Here's how the part is built. I have some questions about the finished solid (model axes, mm). Coordinates: 2 decimals unless noted, no trailing zeros. Order: outer loops, then holes, each group sorted by start corner. A loop starts at its lowest first (then second) coordinate and runs counter-clockwise, first axis right, second up. Notation, with made-up numbers: M 58.5,38 L 93.5,38 A12 cw 93.5,58 Z; hole C 74,46 d1. An arc over 180 degrees is marked long. Answer as CSV lines item,"result". Start each with the question number.
```python
from build123d import *

# Parameters (mm, degrees)
SKETCH_1_W      = 18.84
SKETCH_1_H      = 18.84
EXTRUDE_1_DEPTH = 18.84
FILLET_1_R      = 1
FILLET_2_R      = 3


with BuildPart() as part:
    # 草图1 → 凸台-拉伸1 (new body)
    with BuildSketch(Plane(origin=(0, 0, 0), x_dir=(1, 0, 0), z_dir=(0, 1, 0))):
        Rectangle(SKETCH_1_W, SKETCH_1_H)
    extrude(amount=EXTRUDE_1_DEPTH)

    # 圆角1
    fillet_1_edges = [part.edges().sort_by_distance(p)[0] for p in [
        (0, 18.84, 9.42),
    ]]
    fillet(fillet_1_edges, radius=FILLET_1_R)

    # 圆角2
    fillet_2_edges = [part.edges().sort_by_distance(p)[0] for p in [
        (-9.42, 0, 0),
        (9.42, 0, 0),
        (-9.42, 9.42, -9.42),
        (9.42, 9.42, -9.42),
    ]]
    fillet(fillet_2_edges, radius=FILLET_2_R)


solid = part.part
```
1) Suppose I cut it at B-B on y = 2. Please give me the cut outline in (x, z).
2) Will this pin go through, and if not, where does the flat tip stop? pin 1 Ø6 at (y, z) = (2, -6) entering from -X.
3) I need wall thicknesses on line 1 (Z direction, x = -6.5, y = 2.5); line 2 (X direction, y = 8, z = -7.25); line 3 (Z direction, x = -7.75, y = 7.75). Which ranges of each line are inside material? Lowest first, please. Write a range as [from, to].
4) Suppose I cut it at A-A on x = 7.5. Please give me the cut outline in (y, z), plus the area to 3 significant figures.
Output:
1,outline,"M -9.25,-7.42 A3 ccw -6.42,-9.42 L 6.42,-9.42 A3 ccw 9.25,-7.42 L 9.25,9.42 L -9.25,9.42 Z"
2,pin 1,"x = -9.42"
3,line 1,"[-9.42, 9.42]"
3,line 2,"[-9.3, 9.3]"
3,line 3,"[-9.11, 9.42]"
4,outline,"M 0.2,-9.22 L 18.84,-9.22 L 18.84,8.42 A1 ccw 17.84,9.42 L 0.2,9.42 Z"
4,area,"347 mm²"
